Geometry: final body of the model. Coordinates: model frame, mm. Face numbers are marked on the shaded views. A direction names the side the tool comes from. Coordinates: 2 decimals unless noted, no trailing zeros. Write each loop counter-clockwise with the first axis right and the second up, starting at its lowest first coordinate (ties: lowest second). Pieces come first, ordered by that corner, then holes. Notation, with made-up numbers: (25.5, 78.5) - (57.5, 78.5) arc R23 cw to (57.5, 117.5) - close; hole circle Ø2 at (34, -7.5). An arc over 180 degrees is marked (long way). Answer as a JSON object with one key per item and string values. Group by question number.
Item 1: Mould query, pull axis Z, two halves, no side actions, for the marked faces 1, 2 and 3. Classes: pulls with the +Z half, pulls with the -Z half, needs draft (parallel to the pull), parting line crosses it, or undercut.
Item 2: First-contact query: pin 1 Ø8 at (x, z) = (10, -3.5) entering from +Y; pin 2 Ø10 at (x, z) = (7.5, -13.5) entering from +Y; pin 3 Ø18 at (x, z) = (0, 10.28) entering from -Y. Flat tips, straight axial feed; report the tip coordinate or a pass-through.
Item 3: Section A-A on x = 0. Return loops of the section in (y, z).
Item 4: Section B-B on y = -97.5. Return loops of the section in (x, z), and give its area (3 significant figures).
Item 5: Set-up query: the marked faces 4 and 5. Return all of +Z, -Z, +X, -X, +Y, -Y with unobstructed straight access to the full face (end or side cutting, diameter ignored); none if empty.
Item 6: Line query: line 1 along Z through (x, y) = (0, -16); line 2 along Z through (x, y) = (-13, -93); line 3 along Z through (x, y) = (8.5, -11). Output: solid intervals per line, ascending. Write a range as from..to.
```python
from build123d import *

# Parameters (mm, degrees)
F0_R     = 15
F1_DEPTH = 20
F2_W     = 60
F2_H     = 15
F3_DEPTH = 100
F4_SIZE  = 10


with BuildPart() as f1:
    # F0 (on Front) → F1 (new body)
    with BuildSketch(Plane.XZ):
        with BuildLine():
            Line((-30, -49.717317), (30, -49.717317))
            Line((30, -49.717317), (30, 10.282683))
            ThreePointArc((30, 10.282683), (0, 40.282683), (-30, 10.282683))
            Line((-30, 10.282683), (-30, -49.717317))
        make_face()
        with Locations((0, 10.282683)):
            Circle(F0_R, mode=Mode.SUBTRACT)
    extrude(amount=F1_DEPTH)

    # F2 (on face) → F3 (join)
    with BuildSketch(Plane.XZ.offset(20)):
        with Locations((0, -42.217317)):
            Rectangle(F2_W, F2_H)
    extrude(amount=F3_DEPTH)

    # F4
    f4_edges = [f1.edges().sort_by_distance(p)[0] for p in [
        (-15, 0, 10.282683),
    ]]
    chamfer(f4_edges, length=F4_SIZE)


solid = f1.part
```
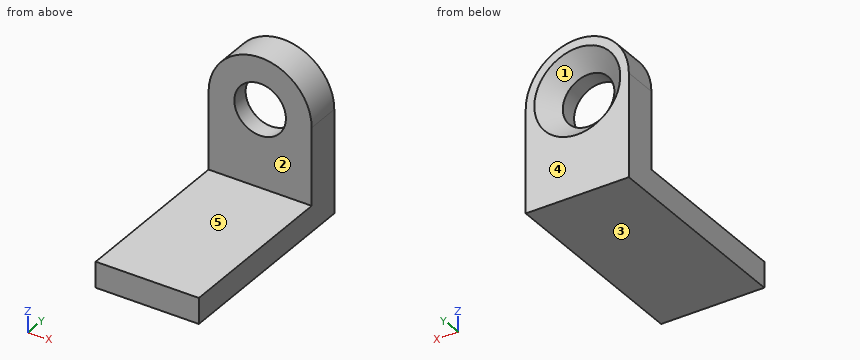
Checks:
{
 "1": {"face 1": "undercut", "face 2": "needs draft", "face 3": "pulls with the -Z half"},
 "2": {"pin 1": "y = -3.97", "pin 2": "y = 0", "pin 3": "through"},
 "3": {"outline": "(-120, -49.72) - (0, -49.72) - (0, -14.72) - (-10, -4.72) - (-20, -4.72) - (-20, -34.72) - (-120, -34.72) - close; (-20, 25.28) - (-10, 25.28) - (0, 35.28) - (0, 40.28) - (-20, 40.28) - close"},
 "4": {"outline": "(-30, -49.72) - (30, -49.72) - (30, -34.72) - (-30, -34.72) - close", "area": "900 mm^2"},
 "5": {"face 4": "+Z, -Z, +X, -X, +Y", "face 5": "+Z, +X, -X, -Y"},
 "6": {"line 1": "-49.72..-4.72, 25.28..40.28", "line 2": "-49.72..-34.72", "line 3": "-49.72..-2.08, 22.64..39.05"}
}
